```python
from build123d import *

# Parameters (mm, degrees)
BOSS_EXTRUDE1_DEPTH = 25.4
SKETCH2_W           = 25.4
SKETCH2_H           = 25.4
BOSS_EXTRUDE2_DEPTH = 609.6
SKETCH3_R           = 38.1
CUT_EXTRUDE1_DEPTH  = 609.6


with BuildPart() as part:
    # Sketch1 → Boss-Extrude1 (new body)
    with BuildSketch(Plane(origin=(0, 0, 0), x_dir=(0, 0, -1), z_dir=(1, 0, 0))):
        with BuildLine():
            Line((0, 0), (-304.8, 0))
            ThreePointArc((-304.8, 0), (-215.526146906, -215.526146906), (0, -304.8))
            Line((0, -304.8), (0, 0))
        make_face()
    boss_extrude1 = extrude(amount=BOSS_EXTRUDE1_DEPTH)

    # Sketch2 → Boss-Extrude2 (add)
    with BuildSketch(Plane(origin=(25.4, 0, 0), x_dir=(0, 0, -1), z_dir=(1, 0, 0))):
        with BuildLine():
            Line((-304.8, 0), (-287.848767292, 0))
            ThreePointArc((-287.848767292, 0), (-226.698239846, -177.38325987), (-69.22826613, -279.4))
            Line((-69.22826613, -279.4), (-69.22826613, -296.834107152))
            ThreePointArc((-69.22826613, -296.834107152), (-238.750723053, -189.475941063), (-304.8, 0))
        make_face()
        with Locations((-12.7, -12.7)):
            Rectangle(SKETCH2_W, SKETCH2_H)
    boss_extrude2 = extrude(amount=BOSS_EXTRUDE2_DEPTH)

    # Sketch3 → Cut-Extrude1 (cut)
    with BuildSketch(Plane.ZY):
        with Locations((127, -127)):
            Circle(SKETCH3_R)
    cut_extrude1 = extrude(amount=-CUT_EXTRUDE1_DEPTH, mode=Mode.SUBTRACT)

    # Mirror2: Boss-Extrude2 across plane
    add(boss_extrude2.mirror(Plane(origin=(635, 0, 0), x_dir=(0, 0, 1), z_dir=(1, 0, 0))))

    # Mirror3: Boss-Extrude1 across plane
    add(boss_extrude1.mirror(Plane(origin=(635, 0, 0), x_dir=(0, 0, 1), z_dir=(1, 0, 0))))

    # Mirror4: Cut-Extrude1 across plane
    add(cut_extrude1.mirror(Plane(origin=(635, 0, 0), x_dir=(0, 0, 1), z_dir=(1, 0, 0))), mode=Mode.SUBTRACT)


solid = part.part
```
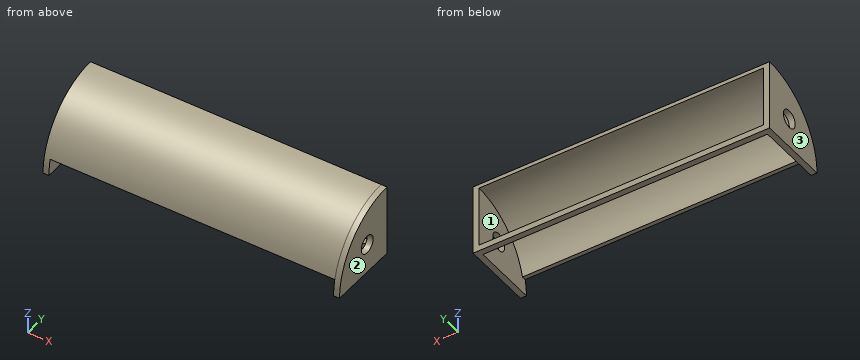
Can you work these out from the model? Positions are in its coordinate system, mm. Face numbers are marked on the shaded views. Coordinates: 2 decimals unless noted, no trailing zeros. Loops run counter-clockwise (first coordinate to the right, second up) from the corner with the lowest first, then second, coordinate; pieces in that order, holes last. Notation, with made-up numbers: (-2, 1) -> (23, 1) arc R17 cw to (23, 24) -> close; hole circle Ø1 at (38, 1). An arc over 180 degrees is marked (long way). Answer as a JSON object with one key per item and string values.
1) Imagine slicing it at B-B (z = 139.5). Please give me the cut outline in (x, y), then the cut area to 3 significant figures.
Results:
{"outline": "(0, -271) -> (1270, -271) -> (1270, -162.99) -> (1244.6, -162.99) -> (1244.6, -251.79) -> (25.4, -251.79) -> (25.4, -162.99) -> (0, -162.99) -> close; (0, -91.01) -> (25.4, -91.01) -> (25.4, 0) -> (0, 0) -> close; (1244.6, -91.01) -> (1270, -91.01) -> (1270, 0) -> (1244.6, 0) -> close", "area": "33,500 mm^2"}
2) For P1, Ø8, axis at x = 954.5, z = 185.5, coming from the +Y side; P2, Ø7.5, axis at x = 821, z = 9.5, coming from the -Y side; P3, Ø5, axis at x = 623.5, y = -287, coming from the -Z side, each with a flat end and sliding along its axis, tell me the tip position at first contact or that it passes through.
Results:
{"P1": "stops at y = -216.67", "P2": "stops at y = -25.4", "P3": "stops at z = 69.23"}
3) Thinking about a two-plate mould opening in X: for the marked faces 1, 2 and 3, which applies, pulls with the +X half, pulls with the -X half, needs draft (parallel to the pull), parting line crosses it, or undercut?
Results:
{"face 1": "undercut", "face 2": "pulls with the +X half", "face 3": "pulls with the -X half"}
4) Imagine slicing it at C-C (y = -261.5). Please give me the cut outline in (x, z).
Results:
{"outline": "(0, 0) -> (25.4, 0) -> (25.4, 120.31) -> (1244.6, 120.31) -> (1244.6, 0) -> (1270, 0) -> (1270, 156.59) -> (0, 156.59) -> close"}
5) Imagine slicing it at D-D (y = -127). Please give me the cut outline in (x, z).
Results:
{"outline": "(0, 0) -> (25.4, 0) -> (25.4, 88.9) -> (0, 88.9) -> close; (0, 165.1) -> (25.4, 165.1) -> (25.4, 258.32) -> (1244.6, 258.32) -> (1244.6, 165.1) -> (1270, 165.1) -> (1270, 277.08) -> (0, 277.08) -> close; (1244.6, 0) -> (1270, 0) -> (1270, 88.9) -> (1244.6, 88.9) -> close"}
6) If I drill on line 1 (X direction, y = -52, z = 51.5); line 2 (Y direction, x = 1251, z = 127); line 3 (Y direction, x = 1169, z = 104), over which ranges is the centre line in solid material (lowest first)?
Results:
{"line 1": "x = 0 to 25.4, 1244.6 to 1270", "line 2": "y = -277.08 to -165.1, -88.9 to 0", "line 3": "y = -286.51 to -268.4"}
7) Imagine slicing it at A-A (x = 818.5). Please give me the cut outline in (y, z).
Results:
{"outline": "(-296.83, 69.23) -> (-279.4, 69.23) arc R287.85 cw to (0, 287.85) -> (0, 304.8) arc R304.8 ccw to start; (-25.4, 0) -> (0, 0) -> (0, 25.4) -> (-25.4, 25.4) -> close"}
